```python
from build123d import *

# Parameters (mm, degrees)
F0_W     = 76.2
F0_H     = 76.2
F1_DEPTH = 38.1
F2_W     = 74.168
F2_H     = 74.168
F3_DEPTH = 36.068
F4_W     = 75.2094
F4_H     = 75.2094
F4_W_2   = 74.168
F4_H_2   = 74.168
F5_DEPTH = 7.62


with BuildPart() as f1:
    # F0 (on Front) → F1 (new body)
    with BuildSketch(Plane.XZ):
        Rectangle(F0_W, F0_H)
    extrude(amount=F1_DEPTH)

    # F2 (on face) → F3 (cut)
    with BuildSketch(Plane(origin=(0, 0, 0), x_dir=(-1, 0, 0), z_dir=(0, 1, 0))):
        Rectangle(F2_W, F2_H)
    extrude(amount=-F3_DEPTH, mode=Mode.SUBTRACT)

    # F4 (on face) → F5 (cut)
    with BuildSketch(Plane(origin=(0, 0, 0), x_dir=(-1, 0, 0), z_dir=(0, 1, 0))):
        Rectangle(F4_W, F4_H)
        Rectangle(F4_W_2, F4_H_2, mode=Mode.SUBTRACT)
    extrude(amount=-F5_DEPTH, mode=Mode.SUBTRACT)


solid = f1.part
```
Read the model definition and answer for the solid it produces. Units are mm, in the model's axes. A direction names the side the tool comes from. Give positions to 0.01 mm unless a question says otherwise; leave off trailing zeros. Write each loop counter-clockwise with the first axis right and the second up, starting at its lowest first coordinate (ties: lowest second). Pieces come first, ordered by that corner, then holes. Notation, with made-up numbers: (1.25, -12.75) -> (59.25, -12.75) arc R22 ccw to (59.25, -4.75) -> close; hole circle Ø6 at (38.25, 43.5). An arc over 180 degrees is marked (long way). Answer as a JSON object with one key per item and string values.
1) A tool of negligible diameter and unlimited length cuts with its end or side. For faces 4 (the flat face through (1, -36.068, 1)), 5 (the flat face through (-1, -19, -38.1)), from which of +Z, -Z, +X, -X, +Y, -Y can it reach the whole face along a straight path? Write none if from no direction.
Findings below:
{"face 4": "+Y", "face 5": "-Z, +X, -X, +Y, -Y"}
2) Straight lines are drawn through the part: probe 1 along Z at (x, y) = (33, -35); probe 2 along X at (y, z) = (-6, 18). For each, find the intervals that lie inside material, in ascending order. Write a range as from..to.
Findings below:
{"probe 1": "z = -38.1..-37.08, 37.08..38.1", "probe 2": "x = -38.1..-37.6, 37.6..38.1"}
3) Section B-B on x = 17 is taken. Write down the section's boundary in (y, z).
Findings below:
{"outline": "(-38.1, -38.1) -> (0, -38.1) -> (0, -37.6) -> (-7.62, -37.6) -> (-7.62, -37.08) -> (-36.07, -37.08) -> (-36.07, 37.08) -> (-7.62, 37.08) -> (-7.62, 37.6) -> (0, 37.6) -> (0, 38.1) -> (-38.1, 38.1) -> close"}
4) A flat-ended cylindrical pin translates along its axis: pin 1 Ø3 at (x, z) = (7, 28) entering from +Y. Find the tip coordinate at first contact, or state that the pin passes through.
Findings below:
{"pin 1": "stops at y = -36.07"}
5) Section C-C on z = -7 is taken. Write down the section's boundary in (x, y), then the cut area to 3 significant figures.
Findings below:
{"outline": "(-38.1, -38.1) -> (38.1, -38.1) -> (38.1, 0) -> (37.6, 0) -> (37.6, -7.62) -> (37.08, -7.62) -> (37.08, -36.07) -> (-37.08, -36.07) -> (-37.08, -7.62) -> (-37.6, -7.62) -> (-37.6, 0) -> (-38.1, 0) -> close", "area": "220 mm^2"}
6) Section D-D on y = -23 is taken. Write down the section's boundary in (x, z).
Findings below:
{"outline": "(-38.1, -38.1) -> (38.1, -38.1) -> (38.1, 38.1) -> (-38.1, 38.1) -> close; hole (-37.08, -37.08) -> (37.08, -37.08) -> (37.08, 37.08) -> (-37.08, 37.08) -> close"}
7) Section A-A on y = -4.5 is taken. Write down the section's boundary in (x, z), then the cut area to 3 significant figures.
Findings below:
{"outline": "(-38.1, -38.1) -> (38.1, -38.1) -> (38.1, 38.1) -> (-38.1, 38.1) -> close; hole (-37.6, -37.6) -> (37.6, -37.6) -> (37.6, 37.6) -> (-37.6, 37.6) -> close", "area": "150 mm^2"}
8) For a pull along X with two mould halves and no side action, classify faces 1 (the flat face through (38.1, -19, -1)), 2 (the flat face through (-1, -38.1, 1)), 3 (the flat face through (1, -22, -37.084)) as pulls with the +X half, pulls with the -X half, needs draft (parallel to the pull), parting line crosses it, or undercut.
Findings below:
{"face 1": "pulls with the +X half", "face 2": "needs draft", "face 3": "undercut"}
